Geometry check sheet. Reference: the model listing, model coordinates, mm. Give positions to 0.01 mm unless a question says otherwise; leave off trailing zeros. Order: outer loops, then holes, each group sorted by start corner. A loop starts at its lowest first (then second) coordinate and runs counter-clockwise, first axis right, second up. Notation, with made-up numbers: M -26.5,61 L 27.5,61 A15 ccw 27.5,83 Z; hole C 51.5,-25.5 d11. An arc over 180 degrees is marked long. Answer as CSV lines item,"result". Start each with the question number.
Autodesk Inventor part; units mm, degrees
ref_plane "Zplus_face" through (0, 0, 1.5875) normal (0, 0, 1) x (1, 0, 0)
ref_plane "Work Plane_ConnX" through (-32, 0, 0) normal (1, 0, 0) x (0, 1, 0)
ref_plane "Work Plane_ConnY" through (0, 0, 0) normal (0, 1, 0) x (-1, 0, 0)
sketch "AL_spacer_contact_Zminus" plane through (0, 0, 0) normal (0, 0, 1) x (1, 0, 0)
  circle A0 centre (39.5, 39.5) radius 3.175
  circle A1 centre (39.5, -39.5) radius 3.175
  circle A2 centre (-39.5, -39.5) radius 3.175
  circle A3 centre (-39.5, 39.5) radius 3.175
  point P0 (0, 0)
  dimension "d228" = 39.5
  dimension "d229" = 39.5
  dimension "d230" = 39.5
  dimension "d231" = 39.5
  dimension "d232" = 39.5
  dimension "d233" = 39.5
  dimension "d234" = 39.5
  dimension "d235" = 39.5
  dimension "d236" = 6.35
sketch "Delrin_stayout_Zminus" plane through (0, 0, 0) normal (0, 0, 1) x (1, 0, 0)
  line L0 (47.5, 39.5) -> (47.5, 31)
  line L1 (47.5, 31) -> (39.5, 31)
  line L2 (39.5, 31) -> (31, 39.5)
  line L3 (31, 39.5) -> (31, 47.5)
  line L4 (31, 47.5) -> (39.5, 47.5)
  line L5 (39.5, 47.5) -> (47.5, 39.5)
  line L6 (-39.5, 47.5) -> (-47.5, 39.5)
  line L7 (-47.5, 39.5) -> (-47.5, 31)
  line L8 (-47.5, 31) -> (-39.5, 31)
  line L9 (-39.5, 31) -> (-31, 39.5)
  line L10 (-31, 39.5) -> (-31, 47.5)
  line L11 (-31, 47.5) -> (-39.5, 47.5)
  line L12 (47.5, -39.5) -> (39.5, -47.5)
  line L13 (39.5, -47.5) -> (31, -47.5)
  line L14 (31, -47.5) -> (31, -39.5)
  line L15 (31, -39.5) -> (39.5, -31)
  line L16 (39.5, -31) -> (47.5, -31)
  line L17 (47.5, -31) -> (47.5, -39.5)
  line L18 (-39.5, -47.5) -> (-47.5, -39.5)
  line L19 (-47.5, -39.5) -> (-47.5, -31)
  line L20 (-47.5, -31) -> (-39.5, -31)
  line L21 (-39.5, -31) -> (-31, -39.5)
  line L22 (-31, -39.5) -> (-31, -47.5)
  line L23 (-31, -47.5) -> (-39.5, -47.5)
  point P0 (0, 0)
  dimension "d243" = 16.5
  dimension "d244" = 8
  dimension "d245" = 8.5
  dimension "d246" = 16.5
  dimension "d247" = 47.5
  dimension "d248" = 47.5
  dimension "d249" = 47.5
  dimension "d250" = 47.5
  dimension "d251" = 47.5
  dimension "d252" = 47.5
  dimension "d253" = 47.5
  dimension "d254" = 47.5
sketch "Nub_stayout_Zminus" plane through (0, 0, 0) normal (0, 0, 1) x (1, 0, 0)
  line L0 (29, 47.5) -> (39.5, 47.5)
  line L1 (39.5, 47.5) -> (47.5, 39.5)
  line L2 (47.5, 39.5) -> (47.5, 29)
  line L3 (47.5, 29) -> (42, 29)
  line L4 (42, 29) -> (42, 40.4125)
  line L5 (40.4125, 42) -> (29, 42)
  line L6 (29, 42) -> (29, 47.5)
  arc A0 (42, 40.4125) -> (40.4125, 42) centre (40.4125, 40.4125) ccw
  line L7 (-29, 47.5) -> (-39.5, 47.5)
  line L8 (-39.5, 47.5) -> (-47.5, 39.5)
  line L9 (-47.5, 39.5) -> (-47.5, 29)
  line L10 (-47.5, 29) -> (-42, 29)
  line L11 (-42, 29) -> (-42, 40.4125)
  line L12 (-40.4125, 42) -> (-29, 42)
  line L13 (-29, 42) -> (-29, 47.5)
  arc A1 (-40.4125, 42) -> (-42, 40.4125) centre (-40.4125, 40.4125) ccw
  line L14 (-47.5, -29) -> (-42, -29)
  line L15 (-42, -29) -> (-42, -40.4125)
  line L16 (-40.4125, -42) -> (-29, -42)
  line L17 (-29, -42) -> (-29, -47.5)
  line L18 (-29, -47.5) -> (-39.5, -47.5)
  line L19 (-39.5, -47.5) -> (-47.5, -39.5)
  line L20 (-47.5, -39.5) -> (-47.5, -29)
  arc A2 (-42, -40.4125) -> (-40.4125, -42) centre (-40.4125, -40.4125) ccw
  line L21 (47.5, -29) -> (42, -29)
  line L22 (42, -29) -> (42, -40.4125)
  line L23 (40.4125, -42) -> (29, -42)
  line L24 (29, -42) -> (29, -47.5)
  line L25 (29, -47.5) -> (39.5, -47.5)
  line L26 (39.5, -47.5) -> (47.5, -39.5)
  line L27 (47.5, -39.5) -> (47.5, -29)
  arc A3 (40.4125, -42) -> (42, -40.4125) centre (40.4125, -40.4125) ccw
  point P0 (0, 0)
  dimension "d255" = 1.5875
  dimension "d256" = 18.5
  dimension "d257" = 8
  dimension "d258" = 5.5
  dimension "d259" = 47.5
  dimension "d260" = 47.5
  dimension "d264" = 1.5875
  dimension "d265" = 47.5
  dimension "d266" = 47.5
  dimension "d267" = 1.5875
  dimension "d268" = 47.5
  dimension "d269" = 47.5
  dimension "d270" = 1.5875
  dimension "d271" = 47.5
  dimension "d272" = 47.5
ref_plane "Zplus_face" through (0, 0, 1.5875) normal (0, 0, 1) x (1, 0, 0)
sketch "AL_spacer_contact_Zplus" plane through (0, 0, 1.5875) normal (0, 0, 1) x (1, 0, 0)
  circle A0 centre (-39.5, 39.5) radius 3.175
  circle A1 centre (-39.5, -39.5) radius 3.175
  circle A2 centre (39.5, -39.5) radius 3.175
  circle A3 centre (39.5, 39.5) radius 3.175
  point P0 (0, 0)
  dimension "d129" = 39.5
  dimension "d130" = 39.5
  dimension "d131" = 39.5
  dimension "d132" = 39.5
  dimension "d133" = 6.35
sketch "Delrin_stayout_Zplus" plane through (0, 0, 1.5875) normal (0, 0, 1) x (1, 0, 0)
  line L0 (47.5, -31) -> (47.5, -39.5)
  line L1 (47.5, -39.5) -> (39.5, -47.5)
  line L2 (39.5, -47.5) -> (31, -47.5)
  line L3 (31, -47.5) -> (31, -39.5)
  line L4 (31, -39.5) -> (39.5, -31)
  line L5 (39.5, -31) -> (47.5, -31)
  line L6 (47.5, 31) -> (47.5, 39.5)
  line L7 (47.5, 39.5) -> (39.5, 47.5)
  line L8 (39.5, 47.5) -> (31, 47.5)
  line L9 (31, 47.5) -> (31, 39.5)
  line L10 (31, 39.5) -> (39.5, 31)
  line L11 (39.5, 31) -> (47.5, 31)
  line L12 (-39.5, 47.5) -> (-47.5, 39.5)
  line L13 (-47.5, 39.5) -> (-47.5, 31)
  line L14 (-47.5, 31) -> (-39.5, 31)
  line L15 (-39.5, 31) -> (-31, 39.5)
  line L16 (-31, 39.5) -> (-31, 47.5)
  line L17 (-31, 47.5) -> (-39.5, 47.5)
  line L18 (-47.5, -39.5) -> (-39.5, -47.5)
  line L19 (-39.5, -47.5) -> (-31, -47.5)
  line L20 (-31, -47.5) -> (-31, -39.5)
  line L21 (-31, -39.5) -> (-39.5, -31)
  line L22 (-39.5, -31) -> (-47.5, -31)
  line L23 (-47.5, -31) -> (-47.5, -39.5)
  point P0 (0, 0)
  dimension "d115" = 16.5
  dimension "d116" = 16.5
  dimension "d117" = 8
  dimension "d118" = 8.5
  dimension "d121" = 47.5
  dimension "d122" = 47.5
  dimension "d123" = 47.5
  dimension "d124" = 47.5
  dimension "d125" = 47.5
  dimension "d126" = 47.5
  dimension "d127" = 47.5
  dimension "d128" = 47.5
sketch "Nub_stayout_Zplus" plane through (0, 0, 1.5875) normal (0, 0, 1) x (1, 0, 0)
  line L0 (47.5, 29) -> (42, 29)
  line L1 (42, 29) -> (42, 40.4125)
  line L2 (40.4125, 42) -> (29, 42)
  line L3 (29, 42) -> (29, 47.5)
  arc A0 (42, 40.4125) -> (40.4125, 42) centre (40.4125, 40.4125) ccw
  line L4 (29, 47.5) -> (39.5, 47.5)
  line L5 (39.5, 47.5) -> (47.5, 39.5)
  line L6 (47.5, 39.5) -> (47.5, 29)
  line L7 (-39.5, 47.5) -> (-29, 47.5)
  line L8 (-29, 47.5) -> (-29, 42)
  line L9 (-29, 42) -> (-40.4125, 42)
  line L10 (-42, 40.4125) -> (-42, 29)
  line L11 (-42, 29) -> (-47.5, 29)
  line L12 (-47.5, 29) -> (-47.5, 39.5)
  line L13 (-47.5, 39.5) -> (-39.5, 47.5)
  arc A1 (-40.4125, 42) -> (-42, 40.4125) centre (-40.4125, 40.4125) ccw
  line L14 (-47.5, -29) -> (-47.5, -39.5)
  line L15 (-47.5, -39.5) -> (-39.5, -47.5)
  line L16 (-39.5, -47.5) -> (-29, -47.5)
  line L17 (-29, -47.5) -> (-29, -42)
  line L18 (-29, -42) -> (-40.4125, -42)
  line L19 (-42, -40.4125) -> (-42, -29)
  line L20 (-42, -29) -> (-47.5, -29)
  arc A2 (-42, -40.4125) -> (-40.4125, -42) centre (-40.4125, -40.4125) ccw
  line L21 (29, -47.5) -> (39.5, -47.5)
  line L22 (39.5, -47.5) -> (47.5, -39.5)
  line L23 (47.5, -39.5) -> (47.5, -29)
  line L24 (47.5, -29) -> (42, -29)
  line L25 (42, -29) -> (42, -40.4125)
  line L26 (40.4125, -42) -> (29, -42)
  line L27 (29, -42) -> (29, -47.5)
  arc A3 (40.4125, -42) -> (42, -40.4125) centre (40.4125, -40.4125) ccw
  point P0 (0, 0)
  dimension "d116" = 16.5
  dimension "d146" = 1.5875
  dimension "d147" = 5.5
  dimension "d149" = 18.5
  dimension "d150" = 8
  dimension "d151" = 47.5
  dimension "d152" = 47.5
  dimension "d153" = 1.5875
  dimension "d154" = 47.5
  dimension "d155" = 47.5
  dimension "d156" = 1.5875
  dimension "d157" = 47.5
  dimension "d158" = 47.5
  dimension "d159" = 1.5875
  dimension "d160" = 47.5
  dimension "d161" = 47.5
sketch "Sketch1" plane through (0, 0, 0) normal (0, 0, 1) x (1, 0, 0)
  line L0 (-47.5, 47.5) -> (47.5, 47.5)
  line L1 (47.5, 47.5) -> (47.5, -47.5)
  line L2 (47.5, -47.5) -> (-47.5, -47.5)
  line L3 (-47.5, -47.5) -> (-47.5, 47.5)
  point P0 (0, 0)
  dimension "d0" = 95
  dimension "d1" = 95
  dimension "d2" = 47.5
  dimension "d3" = 47.5
extrude "Extrusion1" add sketch "Sketch1" along normal blind 1.5875
chamfer "Chamfer2" distance 11 angle 45 4 edges at (-47.5, -47.5, 0.7937) (47.5, -47.5, 0.7937) (47.5, 47.5, 0.7937) (-47.5, 47.5, 0.7937)
ref_plane "Work Plane_ConnX" through (-32, 0, 0) normal (1, 0, 0) x (0, 1, 0)
ref_plane "Work Plane_ConnY" through (0, 0, 0) normal (0, 1, 0) x (-1, 0, 0)
sketch "Sketch9" plane through (0, 0, 1.5875) normal (0, 0, 1) x (1, 0, 0)
  line L0 (47.5, 47.5) -> (47.5, -47.5)
  line L1 (58.5598, -32) -> (-58.5598, -32)
  circle A0 centre (-2.667, -21.9289) radius 0.4445
  circle A1 centre (-2.667, -42.0711) radius 0.4445
  line L2 (0, 26.5598) -> (0, -90.5598) construction
  point P0 (0, 0)
  point P1 (0, -32)
  dimension "d134" = 20.1422
  dimension "d136" = 2.667
  dimension "d138" = 0.889
  dimension "d141" = 180
  dimension "d350" = 32
  dimension "d351" = 0
extrude "Holes_Conn_Zminus" cut sketch "Sketch9" against normal through all
sketch "Sketch22" plane through (0, 0, 1.5875) normal (0, 0, 1) x (1, 0, 0)
  line L0 (47.5, 36.5) -> (47.5, -36.5)
  line L1 (0, -1.0026) -> (0, -62.9974) construction
  line L2 (62.8115, -32) -> (-62.8115, -32)
  circle A0 centre (2.032, -22.7545) radius 0.4445
  circle A1 centre (2.032, -41.2455) radius 0.4445
  point P0 (0, 0)
  point P1 (0, -32)
  dimension "d282" = 180
  dimension "d283" = 18.491
  dimension "d284" = 0.889
  dimension "d285" = 2.032
  dimension "d352" = 32
  dimension "d353" = 0
extrude "Holes_Conn_Zplus" cut sketch "Sketch22" against normal through all
hole "Hole5" at (39.5, 39.5, 1.5875) direction (0, 0, -1) diameter 3.2 end through all
mirror "Mirror5" about plane through (0, 0, 0) normal (1, 0, 0) of "Hole5"
mirror "Mirror6" about plane through (0, 0, 0) normal (0, 1, 0) of "Hole5", "Mirror5"
sketch "Sketch25" plane through (0, 0, 1.5875) normal (0, 0, 1) x (1, 0, 0)
  circle A0 centre (-39.5, -39.5) radius 1.6
  circle A1 centre (39.5, -39.5) radius 1.6
  circle A2 centre (-39.5, 39.5) radius 1.6
  circle A3 centre (39.5, 39.5) radius 1.6
  line L0 (36.5, -47.5) -> (-36.5, -47.5)
  line L1 (0, 0) -> (0, -59.2198)
  line L2 (8, -47.5) -> (8, -15.5)
  line L3 (8, -15.5) -> (-8, -15.5)
  line L4 (-8, -15.5) -> (-8, -47.5)
  line L5 (-8, -47.5) -> (-62.7516, -61.7336)
  line L6 (-62.7516, -61.7336) -> (-64.2933, 68.2222)
  line L7 (-64.2933, 68.2222) -> (58.3572, 62.5728)
  line L8 (58.3572, 62.5728) -> (56.5848, -69.017)
  line L9 (56.5848, -69.017) -> (8, -47.5)
  dimension "d362" = 16
  dimension "d363" = 32
extrude "Extrusion9" [suppressed]
sketch "Sketch26" plane through (0, 0, 1.5875) normal (0, 0, 1) x (1, 0, 0)
  line L0 (-47.5, -36.5) -> (-47.5, 36.5)
  line L1 (36.5, -47.5) -> (-36.5, -47.5)
  line L2 (47.5, 36.5) -> (47.5, -36.5)
  line L3 (-36.5, 47.5) -> (36.5, 47.5)
  line L4 (-47.4469, 47.553) -> (47.5, 47.5) construction
  line L5 (47.5, 47.5) -> (47.4469, -47.553) construction
  line L6 (47.4469, -47.553) -> (-47.5, -47.5) construction
  line L7 (-47.5, -47.5) -> (-47.4469, 47.553) construction
  point P0 (0, 0)
decal "Decal1"
sketch "Sketch27" plane through (0, 0, 0) normal (0, 0, -1) x (-1, 0, 0)
  line L0 (-47.5, 36.5) -> (-47.5, -36.5)
  line L1 (-36.5, -47.5) -> (36.5, -47.5)
  line L2 (47.5, -36.5) -> (47.5, 36.5)
  line L3 (-47.5, 47.5) -> (47.5, 47.5) construction
  line L4 (47.5, 47.5) -> (47.5, -47.5) construction
  line L5 (47.5, -47.5) -> (-47.5, -47.5) construction
  line L6 (-47.5, -47.5) -> (-47.5, 47.5) construction
  point P0 (0, 0)
decal "Decal2"
properties part number "PCB_VUC" material "FR4"
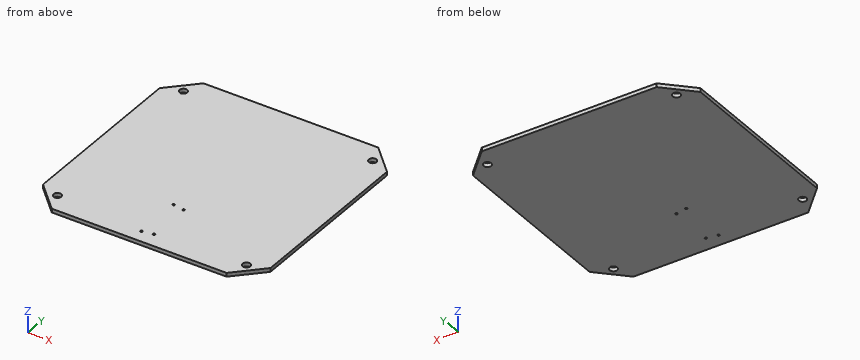
Item 1: Section check C-C on z = 0.25. Give the number of separate pieces and of enclosed holes in the cut face, then the cut area to 3 significant figures.
Item 2: Depth check by flat-ended pin: pin 1 Ø2.5 at (x, y) = (39.5, 39.5) entering from +Z. Enter the tip coordinate at first touch or a pass-through.
Item 3: Section check A-A on x = -39.5. Record the boundary of the cut face in (y, z), then the cut area to 3 significant figures.
Item 4: Scan lines: line 1 along Y through (x, z) = (39.5, 0.7); line 2 along Y through (x, z) = (-40.5, 1.1). Record each from-to range of solid material in increasing order.
Numbers:
1,separate pieces,"1"
1,enclosed holes,"8"
1,area,"8,750 mm2"
2,pin 1,"through"
3,outline,"M -44.5,0 L -41.1,0 L -41.1,1.59 L -44.5,1.59 Z; M -37.9,0 L 37.9,0 L 37.9,1.59 L -37.9,1.59 Z; M 41.1,0 L 44.5,0 L 44.5,1.59 L 41.1,1.59 Z"
3,area,"131 mm2"
4,line 1,"-44.5 to -41.1, -37.9 to 37.9, 41.1 to 44.5"
4,line 2,"-43.5 to -40.75, -38.25 to 38.25, 40.75 to 43.5"
